Can you work these out from the drawing? Everything is in mm from the part's minimum corner. A direction names the side the tool comes from. Round coordinates to 2 decimals unless told otherwise and drop trailing zeros. Write each loop counter-clockwise with the first axis right and the second up, starting at its lowest first coordinate (ties: lowest second). Pieces come first, ordered by that corner, then holes. Notation, with made-up numbers: (76, 7) -> (106, 7) arc R26 ccw to (106, 40) -> close; hole circle Ø11 at (56, -16). An arc over 180 degrees is marked (long way). Write item = value, one per line. Start each with the question number.
1) Imagine slicing it at D-D, the plane y = 65. Please give me the cut outline in (x, z).
2) Imagine slicing it at B-B, the plane z = 3.5. Please give me the cut outline in (x, y).
3) For the marked faces 1 and 2, which set-ups out of +Z, -Z, +X, -X, +Y, -Y let a thin tool reach every point of the face, with its end or its side?
4) I'm going to push flat-ended pins straight in: pin 1 (2 mm diameter, centred on y = 41, z = 2.5, fed in from +X); pin 2 (0.8 mm diameter, centred on x = 2.5, y = 69.5, fed in from -Z); pin 3 (4.5 mm diameter, centred on x = 9, y = 45, fed in from -Z). Where does each tip first touch, or does it pass through?
5) Imagine slicing it at C-C, the plane y = 30. Please give me the cut outline in (x, z), then the cut area to 4 significant figures.
6) Imagine slicing it at A-A, the plane x = 9. Please give me the cut outline in (y, z), then the cut area to 3 significant figures.
7) If I drill on line 1 (Y direction, x = 2.5, z = 4.5); line 2 (Y direction, x = 9, z = 5.75); line 3 (X direction, y = 25, z = 6.35), over which ranges is the centre line in solid material (lowest first)?
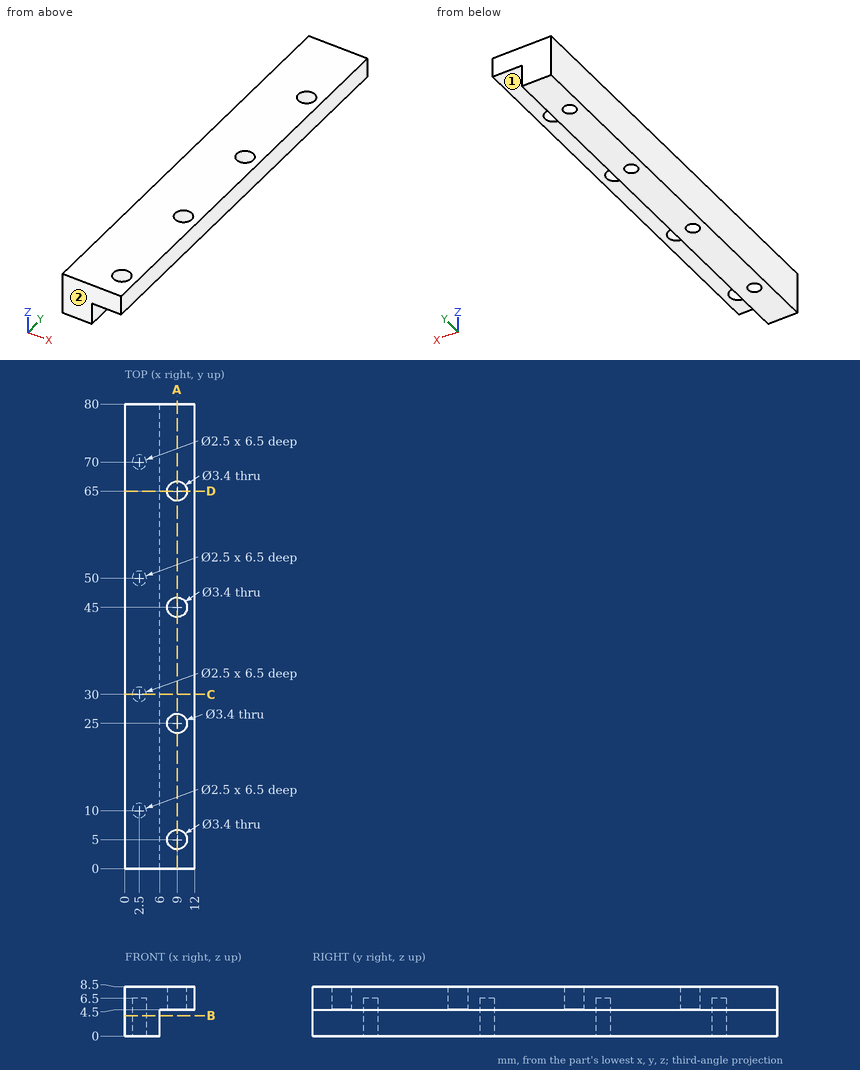
Reported:
q1.outline = (0, 0) -> (6, 0) -> (6, 4.5) -> (7.3, 4.5) -> (7.3, 8.5) -> (0, 8.5) -> close; (10.7, 4.5) -> (12, 4.5) -> (12, 8.5) -> (10.7, 8.5) -> close
q2.outline = (0, 0) -> (6, 0) -> (6, 80) -> (0, 80) -> close; hole circle Ø2.5 at (2.5, 10); hole circle Ø2.5 at (2.5, 30); hole circle Ø2.5 at (2.5, 50); hole circle Ø2.5 at (2.5, 70)
q3.face_1 = -Z, +X, +Y, -Y
q3.face_2 = +Z, -Z, +X, -X, -Y
q4.pin_1 = 6
q4.pin_2 = 6.5
q4.pin_3 = 4.5
q5.outline = (0, 0) -> (1.25, 0) -> (1.25, 6.5) -> (3.75, 6.5) -> (3.75, 0) -> (6, 0) -> (6, 4.5) -> (12, 4.5) -> (12, 8.5) -> (0, 8.5) -> close
q5.area = 58.75 mm²
q6.outline = (0, 4.5) -> (3.3, 4.5) -> (3.3, 8.5) -> (0, 8.5) -> close; (6.7, 4.5) -> (23.3, 4.5) -> (23.3, 8.5) -> (6.7, 8.5) -> close; (26.7, 4.5) -> (43.3, 4.5) -> (43.3, 8.5) -> (26.7, 8.5) -> close; (46.7, 4.5) -> (63.3, 4.5) -> (63.3, 8.5) -> (46.7, 8.5) -> close; (66.7, 4.5) -> (80, 4.5) -> (80, 8.5) -> (66.7, 8.5) -> close
q6.area = 266 mm²
q7.line_1 = 0 to 8.75, 11.25 to 28.75, 31.25 to 48.75, 51.25 to 68.75, 71.25 to 80
q7.line_2 = 0 to 3.3, 6.7 to 23.3, 26.7 to 43.3, 46.7 to 63.3, 66.7 to 80
q7.line_3 = 0 to 7.3, 10.7 to 12
